```python
from build123d import *

# Parameters (mm, degrees)
SKETCH1_W               = 5
SKETCH1_H               = 5
SKETCH1_R               = 0.95
CENTER_DEPTH            = 1.3
RIGHTSIDE_START         = 1.3
SKETCH1_2_W             = 5
SKETCH1_2_H             = 5
SKETCH1_2_R             = 0.95
RIGHTSIDE_DEPTH         = 1.2
LEFTSIDE_START          = -1.3
SKETCH1_3_W             = 5
SKETCH1_3_H             = 5
SKETCH1_3_R             = 0.95
LEFTSIDE_DEPTH          = 1.2
SKETCH3_W               = 5
SKETCH3_H               = 5
BOSS_EXTRUDE4_DEPTH     = 47.5
CUT_EXTRUDE1_DEPTH      = 5
CIRPATTERN2_COUNT       = 6
CIRPATTERN3_COUNT       = 3
CIRPATTERN4_START       = -1.3
CIRPATTERN4_OUTLINE_W   = 5
CIRPATTERN4_OUTLINE_H   = 5
CIRPATTERN4_OUTLINE_R   = 0.95
CIRPATTERN4_DEPTH       = 2.6
CIRPATTERN4_START_2     = -44.601270189
CIRPATTERN4_2_OUTLINE_W = 5
CIRPATTERN4_2_OUTLINE_H = 5
CIRPATTERN4_2_OUTLINE_R = 0.95
CIRPATTERN4_2_DEPTH     = 2.6
CIRPATTERN4_3_OUTLINE_W = 5
CIRPATTERN4_3_OUTLINE_H = 5
CIRPATTERN4_3_OUTLINE_R = 0.95
CIRPATTERN4_3_DEPTH     = 2.6
SKETCH5_W               = 5
SKETCH5_H               = 2.6
CUT_EXTRUDE2_DEPTH      = 5


# Read off the part's stored shape, not the designer's step: CirPattern4
with BuildPart() as part:
    # Sketch1 → Center (new, symmetric)
    with BuildSketch(Plane(origin=(0, 0, 0), x_dir=(1, 0, 0), z_dir=(0, 1, 0))):
        Rectangle(SKETCH1_W, SKETCH1_H)
        with Locations(Location((0, 0, 0), (0, 0, 270))):
            Circle(SKETCH1_R, mode=Mode.SUBTRACT)
    extrude(amount=CENTER_DEPTH, both=True)

    # Sketch5 → Cut-Extrude2 (cut)
    with BuildSketch(Plane(origin=(2.5, 0, 0), x_dir=(0, 0, -1), z_dir=(1, 0, 0))):
        Rectangle(SKETCH5_W, SKETCH5_H)
    extrude(amount=-CUT_EXTRUDE2_DEPTH, mode=Mode.SUBTRACT)


with BuildPart() as body_2:
    # Sketch1<2> → RightSide (new body)
    with BuildSketch(Plane(origin=(0, 0, 0), x_dir=(1, 0, 0), z_dir=(0, 1, 0)).offset(RIGHTSIDE_START)):
        Rectangle(SKETCH1_2_W, SKETCH1_2_H)
        with Locations(Location((0, 0, 0), (0, 0, 270))):
            Circle(SKETCH1_2_R, mode=Mode.SUBTRACT)
    extrude(amount=RIGHTSIDE_DEPTH)


with BuildPart() as body_3:
    # Sketch1<3> → LeftSide (new body)
    with BuildSketch(Plane(origin=(0, 0, 0), x_dir=(1, 0, 0), z_dir=(0, 1, 0)).offset(LEFTSIDE_START)):
        Rectangle(SKETCH1_3_W, SKETCH1_3_H)
        with Locations(Location((0, 0, 0), (0, 0, 270))):
            Circle(SKETCH1_3_R, mode=Mode.SUBTRACT)
    extrude(amount=-LEFTSIDE_DEPTH)


with BuildPart() as body_4:
    # Sketch3 → Boss-Extrude4 (new body)
    with BuildSketch(Plane.ZY.offset(2.5)):
        Rectangle(SKETCH3_W, SKETCH3_H)
    extrude(amount=BOSS_EXTRUDE4_DEPTH)

    # Sketch4 → Cut-Extrude1 (cut)
    with BuildSketch(Plane.XY.offset(-2.5)):
        Polygon((-50, 0), (-50, -2.5), (-45.669872981, -2.5), align=None)
        Polygon((-50, 2.5), (-50, 0), (-45.669872981, 2.5), align=None)
    extrude(amount=CUT_EXTRUDE1_DEPTH, mode=Mode.SUBTRACT)


with BuildPart() as cirpattern2_1:
    # CirPattern2: pattern copy
    add(body_4.part.rotate(Axis((-50, 0, 0), (0, 0, 1)), 1 * 360 / CIRPATTERN2_COUNT))


with BuildPart() as cirpattern2_2:
    # CirPattern2: pattern copy
    add(body_4.part.rotate(Axis((-50, 0, 0), (0, 0, 1)), 2 * 360 / CIRPATTERN2_COUNT))


with BuildPart() as cirpattern2_3:
    # CirPattern2: pattern copy
    add(body_4.part.rotate(Axis((-50, 0, 0), (0, 0, 1)), 3 * 360 / CIRPATTERN2_COUNT))


with BuildPart() as cirpattern2_4:
    # CirPattern2: pattern copy
    add(body_4.part.rotate(Axis((-50, 0, 0), (0, 0, 1)), 4 * 360 / CIRPATTERN2_COUNT))


with BuildPart() as cirpattern2_5:
    # CirPattern2: pattern copy
    add(body_4.part.rotate(Axis((-50, 0, 0), (0, 0, 1)), 5 * 360 / CIRPATTERN2_COUNT))


with BuildPart() as cirpattern3_1:
    # CirPattern3: pattern copy
    add(body_3.part.rotate(Axis((-50, 0, 0), (0, 0, 1)), 1 * 360 / CIRPATTERN3_COUNT))


with BuildPart() as cirpattern3_2:
    # CirPattern3: pattern copy
    add(body_3.part.rotate(Axis((-50, 0, 0), (0, 0, 1)), 2 * 360 / CIRPATTERN3_COUNT))


with BuildPart() as cirpattern3_3:
    # CirPattern3: pattern copy
    add(body_2.part.rotate(Axis((-50, 0, 0), (0, 0, 1)), 1 * 360 / CIRPATTERN3_COUNT))


with BuildPart() as cirpattern3_4:
    # CirPattern3: pattern copy
    add(body_2.part.rotate(Axis((-50, 0, 0), (0, 0, 1)), 2 * 360 / CIRPATTERN3_COUNT))


with BuildPart() as body_14:
    # CirPattern4 outline → CirPattern4 (new body)
    with BuildSketch(Plane(origin=(0, 0, 0), x_dir=(1, 0, 0), z_dir=(0, 1, 0)).offset(CIRPATTERN4_START)):
        with Locations((-100, 0)):
            Rectangle(CIRPATTERN4_OUTLINE_W, CIRPATTERN4_OUTLINE_H)
        with Locations((-100, 0)):
            Circle(CIRPATTERN4_OUTLINE_R, mode=Mode.SUBTRACT)
    extrude(amount=CIRPATTERN4_DEPTH)


with BuildPart() as body_15:
    # CirPattern4 2 outline → CirPattern4 2 (new body)
    with BuildSketch(Plane(origin=(0, 0, 0), x_dir=(0.5000000000000098, -0.8660254037844329, 0), z_dir=(0.8660254037844329, 0.50000000000001, 0)).offset(CIRPATTERN4_START_2)):
        with Locations((25, 0)):
            Rectangle(CIRPATTERN4_2_OUTLINE_W, CIRPATTERN4_2_OUTLINE_H)
        with Locations((25, 0)):
            Circle(CIRPATTERN4_2_OUTLINE_R, mode=Mode.SUBTRACT)
    extrude(amount=CIRPATTERN4_2_DEPTH)


with BuildPart() as body_16:
    # CirPattern4 3 outline → CirPattern4 3 (new body)
    with BuildSketch(Plane(origin=(0, 0, 0), x_dir=(0.49999999999999767, 0.86602540378444, 0), z_dir=(0.8660254037844399, -0.49999999999999795, 0)).offset(CIRPATTERN4_START_2)):
        with Locations((25, 0)):
            Rectangle(CIRPATTERN4_3_OUTLINE_W, CIRPATTERN4_3_OUTLINE_H)
        with Locations((25, 0)):
            Circle(CIRPATTERN4_3_OUTLINE_R, mode=Mode.SUBTRACT)
    extrude(amount=CIRPATTERN4_3_DEPTH)


with BuildPart() as cirpattern3_1_1:
    add(cirpattern3_1.part)

    # Combine1: union CirPattern3_3, CirPattern2_2, body 16, CirPattern2_1, body 3, body 2, body 4
    add(cirpattern3_3.part)
    add(cirpattern2_2.part)
    add(body_16.part)
    add(cirpattern2_1.part)
    add(body_3.part)
    add(body_2.part)
    add(body_4.part)

    # Combine3: cut CirPattern2_5, CirPattern3_2, body 15, CirPattern2_4, CirPattern3_4, CirPattern2_3, body 14
    add(cirpattern2_5.part, mode=Mode.SUBTRACT)
    add(cirpattern3_2.part, mode=Mode.SUBTRACT)
    add(body_15.part, mode=Mode.SUBTRACT)
    add(cirpattern2_4.part, mode=Mode.SUBTRACT)
    add(cirpattern3_4.part, mode=Mode.SUBTRACT)
    add(cirpattern2_3.part, mode=Mode.SUBTRACT)
    add(body_14.part, mode=Mode.SUBTRACT)


solid = cirpattern3_1_1.part
```
Verification items for the finished model (mm, model axes). A direction names the side the tool comes from. Round coordinates to 2 decimals unless told otherwise and drop trailing zeros. Write each loop counter-clockwise with the first axis right and the second up, starting at its lowest first coordinate (ties: lowest second). Pieces come first, ordered by that corner, then holes. Notation, with made-up numbers: (84, 70.25) -> (126, 70.25) arc R19 cw to (126, 104.25) -> close; hole circle Ø3 at (47.5, 41). An arc over 180 degrees is marked (long way). Write each question's results on one line, items separated by ' | '.
Q1. Access from +Z, -Z, +X, -X, +Y, -Y to the whole of each face (thin tool, end or side, straight path). Record for faces 5 (the face through (-26.7, 42.96, 0.04)), 6 (the face through (1.1, -1.3, 0)), 7 (the face through (-23.77, 45.48, -0.03)), 8 (the face through (-73.683, 44.803, -0.7)), 9 (the face through (-73.766, 41.127, -0.035)).
Derived:
face 5: +Z, -Z, +Y | face 6: +Z, -Z, +X | face 7: +Z, -Z, +X, +Y | face 8: none | face 9: +Z, -Z
Q2. Sectioned sample at D-D, the plane x = -11.5. Record the boundary of the cut face in (y, z).
Derived:
outline: (-2.5, -2.5) -> (2.5, -2.5) -> (2.5, 2.5) -> (-2.5, 2.5) -> close
Q3. Sectioned sample at B-B, the plane y = 28. Record the boundary of the cut face in (x, z).
Derived:
outline: (-69.05, -2.5) -> (-63.28, -2.5) -> (-63.28, 2.5) -> (-69.05, 2.5) -> close; (-36.72, -2.5) -> (-30.95, -2.5) -> (-30.95, 2.5) -> (-36.72, 2.5) -> close
Q4. Sectioned sample at A-A, the plane x = 0. Record the boundary of the cut face in (y, z), and give its area (3 significant figures).
Derived:
outline: (-2.5, -2.5) -> (-1.3, -2.5) -> (-1.3, -0.95) -> (-2.5, -0.95) -> close; (-2.5, 0.95) -> (-1.3, 0.95) -> (-1.3, 2.5) -> (-2.5, 2.5) -> close; (1.3, -2.5) -> (2.5, -2.5) -> (2.5, -0.95) -> (1.3, -0.95) -> close; (1.3, 0.95) -> (2.5, 0.95) -> (2.5, 2.5) -> (1.3, 2.5) -> close | area: 7.44 mm²
Q5. Go/stop test with flat-tipped pins: pin 1 Ø3 at (x, z) = (-42.5, 0) entering from +Y; pin 2 Ø2.5 at (x, z) = (-1, -1) entering from +Y; pin 3 Ø2 at (y, z) = (17.5, 0.5) entering from +X; pin 4 Ø5 at (x, y) = (-65, 11.5) entering from +Z. Record where each tip stops, or that it passes through.
Derived:
pin 1: stops at y = 20.59 | pin 2: stops at y = 2.5 | pin 3: stops at x = -36.43 | pin 4: passes through
Q6. Draft check along Z on faces 1 (the face through (-41, 15, 2.5)), 2 (the face through (-25.49, 42.49, 0.04)), 3 (the face through (-0.36, 1.89, 0.88)), 4 (the face through (-39.06, 23.95, -0.03)). Enter one of: released by +Z, released by -Z, zero draft, split by the parting line, or undercut.
Derived:
face 1: released by +Z | face 2: undercut | face 3: undercut | face 4: zero draft
Q7. Thickness scan on probe 1 along X at (y, z) = (41, -1.8); probe 2 along Z at (x, y) = (0, -1.9); probe 3 along X at (y, z) = (1.7, 0). Record the ranges inside material, lowest first.
Derived:
probe 1: x = -76.56 to -75.17, -73.99 to -70.78, -29.22 to -24.83 | probe 2: z = -2.5 to -0.95, 0.95 to 2.5 | probe 3: x = -52.94 to -0.95, 0.95 to 2.5
Q8. Sectioned sample at C-C, the plane x = -44. Record the boundary of the cut face in (y, z), and give its area (3 significant figures).
Derived:
outline: (-2.5, -2.5) -> (2.5, -2.5) -> (2.5, 2.5) -> (-2.5, 2.5) -> close; (5.39, -2.5) -> (15.39, -2.5) -> (15.39, 2.5) -> (5.39, 2.5) -> close | area: 75.0 mm²
